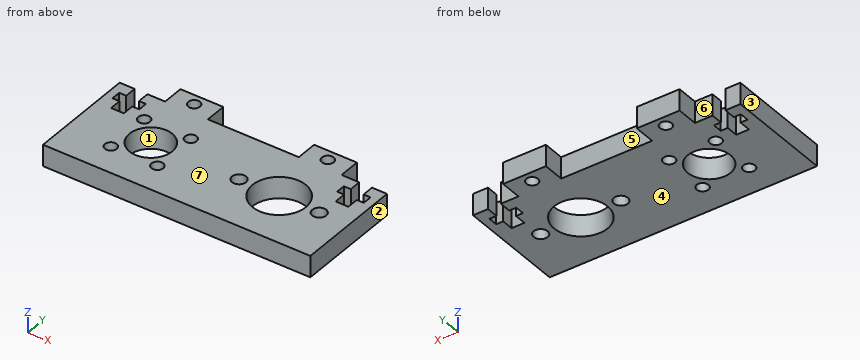
from build123d import *

# Parameters (mm, degrees)
SKETCH1_W           = 39.6875
SKETCH1_H           = 31.75
BOSS_EXTRUDE1_DEPTH = 6.35
SKETCH2_R           = 6.35
SKETCH2_R_2         = 1.7526
CUT_EXTRUDE1_DEPTH  = 6.35
CUT_EXTRUDE4_DEPTH  = 6.35
SKETCH4_W           = 12.7
SKETCH4_H           = 6.35
SKETCH4_R           = 1.7526
BOSS_EXTRUDE2_DEPTH = 6.35
SKETCH5_R           = 7.9375
SKETCH5_R_2         = 2.0828
CUT_EXTRUDE3_DEPTH  = 6.35


with BuildPart() as part:
    # Sketch1 → Boss-Extrude1 (new body)
    with BuildSketch(Plane.XY):
        with Locations((-19.84375, 0)):
            Rectangle(SKETCH1_W, SKETCH1_H)
    boss_extrude1 = extrude(amount=BOSS_EXTRUDE1_DEPTH)

    # Sketch2 → Cut-Extrude1 (cut)
    with BuildSketch(Plane.XY.offset(6.35)):
        with Locations((-19.05, 0)):
            Circle(SKETCH2_R)
        with Locations((-25.964797213, 6.914797213)):
            Circle(SKETCH2_R_2)
        with Locations((-12.135202787, 6.914797213)):
            Circle(SKETCH2_R_2)
        with Locations((-12.135202787, -6.914797213)):
            Circle(SKETCH2_R_2)
        with Locations((-25.964797213, -6.914797213)):
            Circle(SKETCH2_R_2)
    extrude(amount=-CUT_EXTRUDE1_DEPTH, mode=Mode.SUBTRACT)

    # Sketch3 → Cut-Extrude4 (cut)
    with BuildSketch(Plane.XY.offset(6.35)):
        Polygon((-35.23615, 6.096), (-31.43885, 6.096), (-31.43885, 9.5964375), (-29.36875, 9.5964375), (-29.36875, 12.3745625), (-31.43885, 12.3745625), (-31.43885, 15.875), (-35.23615, 15.875), (-35.23615, 12.3745625), (-37.30625, 12.3745625), (-37.30625, 9.5964375), (-35.23615, 9.5964375), align=None)
    cut_extrude4 = extrude(amount=-CUT_EXTRUDE4_DEPTH, mode=Mode.SUBTRACT)

    # Sketch4 → Boss-Extrude2 (add)
    with BuildSketch(Plane.XY.offset(6.35)):
        with Locations((-19.84375, 19.05)):
            Rectangle(SKETCH4_W, SKETCH4_H)
        with Locations((-19.84375, 19.05)):
            Circle(SKETCH4_R, mode=Mode.SUBTRACT)
    boss_extrude2 = extrude(amount=-BOSS_EXTRUDE2_DEPTH)

    # Mirror1: Boss-Extrude1, Cut-Extrude4, Boss-Extrude2 across plane
    add(boss_extrude1.mirror(Plane(origin=(0, -15.875, 6.35), x_dir=(0, 0, 1), z_dir=(-1, 0, 0))))
    add(cut_extrude4.mirror(Plane(origin=(0, -15.875, 6.35), x_dir=(0, 0, 1), z_dir=(-1, 0, 0))), mode=Mode.SUBTRACT)
    add(boss_extrude2.mirror(Plane(origin=(0, -15.875, 6.35), x_dir=(0, 0, 1), z_dir=(-1, 0, 0))))

    # Sketch5 → Cut-Extrude3 (cut)
    with BuildSketch(Plane.XY.offset(6.35)):
        with Locations((19.05, 0)):
            Circle(SKETCH5_R)
        with Locations((7.14375, 0)):
            Circle(SKETCH5_R_2)
        with Locations((30.95625, 0)):
            Circle(SKETCH5_R_2)
    extrude(amount=-CUT_EXTRUDE3_DEPTH, mode=Mode.SUBTRACT)


solid = part.part
Verification items for the finished model (mm, model axes). Face numbers are marked on the shaded views. A direction names the side the tool comes from. Round coordinates to 2 decimals unless told otherwise and drop trailing zeros. Order: outer loops, then holes, each group sorted by start corner. A loop starts at its lowest first (then second) coordinate and runs counter-clockwise, first axis right, second up. Notation, with made-up numbers: (80, 85) -> (119, 85) arc R37 cw to (119, 123) -> close; hole circle Ø1 at (-7, -6.75). An arc over 180 degrees is marked (long way). Put each result on its own line as item: value.
1) Set-up check for the marked faces 5, 6 and 7: record each of +Z, -Z, +X, -X, +Y, -Y from which the full face is reachable in a straight line by a thin tool's end or side.
Final values:
face 5: +Z, -Z, +Y
face 6: +Z, -Z, -X, +Y
face 7: +Z, +X, -X, +Y, -Y
2) Material ranges on line 1 (Y direction, x = 19.5, z = 4.75) (3 decimals); line 2 (X direction, y = 18, z = 3); line 3 (X direction, y = 11.5, z = 2.5), recorded low to high.
Final values:
line 1: y = -15.875 to -7.925, 7.925 to 17.331, 20.769 to 22.225
line 2: x = -26.19 to -21.25, -18.44 to -13.49, 13.49 to 18.44, 21.25 to 26.19
line 3: x = -39.69 to -37.31, -29.37 to 29.37, 37.31 to 39.69
3) Depth check by flat-ended pin: pin 1 (3 mm diameter, centred on x = -12.14, y = 6.91, fed in from +Z); pin 2 (5.5 mm diameter, centred on x = -25.96, y = 6.91, fed in from +Z); pin 3 (1.7 mm diameter, centred on x = 30, z = 2, fed in from +Y) (3 decimals); pin 4 (3 mm diameter, centred on y = 18.5, z = 3, fed in from -X). Enter the tip coordinate at first touch or a pass-through.
Final values:
pin 1: passes through
pin 2: stops at z = 6.35
pin 3: stops at y = 15.875
pin 4: stops at x = -26.19
4) Section check D-D (x = 6). Record the cut outline in (y, z) (3 decimals).
Final values:
outline: (-15.875, 0) -> (-1.741, 0) -> (-1.741, 6.35) -> (-15.875, 6.35) -> close; (1.741, 0) -> (15.875, 0) -> (15.875, 6.35) -> (1.741, 6.35) -> close
5) Section check A-A (y = 19.05). Record the cut outline in (x, z).
Final values:
outline: (-26.19, 0) -> (-21.6, 0) -> (-21.6, 6.35) -> (-26.19, 6.35) -> close; (-18.09, 0) -> (-13.49, 0) -> (-13.49, 6.35) -> (-18.09, 6.35) -> close; (13.49, 0) -> (18.09, 0) -> (18.09, 6.35) -> (13.49, 6.35) -> close; (21.6, 0) -> (26.19, 0) -> (26.19, 6.35) -> (21.6, 6.35) -> close
6) Section check C-C (y = 0). Record the cut outline in (x, z).
Final values:
outline: (-39.69, 0) -> (-25.4, 0) -> (-25.4, 6.35) -> (-39.69, 6.35) -> close; (-12.7, 0) -> (5.06, 0) -> (5.06, 6.35) -> (-12.7, 6.35) -> close; (9.23, 0) -> (11.11, 0) -> (11.11, 6.35) -> (9.23, 6.35) -> close; (26.99, 0) -> (28.87, 0) -> (28.87, 6.35) -> (26.99, 6.35) -> close; (33.04, 0) -> (39.69, 0) -> (39.69, 6.35) -> (33.04, 6.35) -> close
7) Mould release check, pull along X, two halves, no side actions. Record for the marked faces 1, 2, 3 and 4: +X half, -X half, draft (parallel to the pull), parting line (faces both ways), or undercut.
Final values:
face 1: undercut
face 2: +X half
face 3: -X half
face 4: draft
8) Section check B-B (x = -19.05). Record the cut outline in (y, z) (3 decimals), then the cut area to 3 significant figures.
Final values:
outline: (-15.875, 0) -> (-6.35, 0) -> (-6.35, 6.35) -> (-15.875, 6.35) -> close; (6.35, 0) -> (17.487, 0) -> (17.487, 6.35) -> (6.35, 6.35) -> close; (20.613, 0) -> (22.225, 0) -> (22.225, 6.35) -> (20.613, 6.35) -> close
area: 141 mm^2
